CAD build for the part. Positions are in the model's coordinates, mm. A direction names the side the tool comes from. Coordinates: 2 decimals unless noted, no trailing zeros. Order: outer loops, then holes, each group sorted by start corner. A loop starts at its lowest first (then second) coordinate and runs counter-clockwise, first axis right, second up. Notation, with made-up numbers: (-1.5, -28.5) - (16.5, -28.5) arc R26 ccw to (16.5, 6.5) - close; hole circle Ø11 at (-12, 34). An arc over 180 degrees is marked (long way). Use one line per item in the form item = value.
```python
from build123d import *

# Parameters (mm, degrees)
F0_R     = 1
F1_DEPTH = 6.35


with BuildPart() as f1:
    # F0 (on Top) → F1 (new body)
    with BuildSketch(Plane.XY):
        with BuildLine():
            Line((-44.45, 22.732547), (-44.45, -22.6289))
            Line((-44.45, -22.6289), (5.08, -22.6289))
            Line((5.08, -22.6289), (5.08, -17.8029))
            Line((5.08, -17.8029), (9.652, -17.8029))
            Line((9.652, -17.8029), (9.652, -22.248723))
            ThreePointArc((9.652, -22.248723), (32.178133, 0.241912), (9.652, 22.732547))
            Line((9.652, 22.732547), (9.652, 17.906547))
            Line((9.652, 17.906547), (5.08, 17.906547))
            Line((5.08, 17.906547), (5.08, 22.732547))
            Line((5.08, 22.732547), (-44.45, 22.732547))
        make_face()
        with Locations((-24.760989, 0)):
            Circle(F0_R, mode=Mode.SUBTRACT)
        with Locations((5.589839, 0)):
            Circle(F0_R, mode=Mode.SUBTRACT)
        with Locations((20.59151, 0)):
            Circle(F0_R, mode=Mode.SUBTRACT)
    extrude(amount=F1_DEPTH)


solid = f1.part
```
Item 1: Drop flat-ended pins along their axis: pin 1 (1.4 mm diameter, centred on y = -20.5, z = 2, fed in from +X); pin 2 (1.5 mm diameter, centred on x = 14.5, z = 2, fed in from -Y); pin 3 (2.5 mm diameter, centred on x = 7, z = 2, fed in from -Y). Give the stop position or say it passes through.
Derived:
pin_1 = 19.89
pin_2 = -21.88
pin_3 = -17.8
Item 2: Drill centre lines: line 1 (X direction, y = 20, z = 4); line 2 (X direction, y = -10.5, z = 3.5); line 3 (X direction, y = 7, z = 0.5). Where is each one in solid material? Low to high. Write a range as [from, to].
Derived:
line_1 = [-44.45, 5.08], [9.65, 20.43]
line_2 = [-44.45, 29.45]
line_3 = [-44.45, 31.14]
Item 3: Cut at B-B, the plane y = 0. Write the cut outline in (x, z).
Derived:
outline = (-44.45, 0) - (-25.76, 0) - (-25.76, 6.35) - (-44.45, 6.35) - close; (-23.76, 0) - (4.59, 0) - (4.59, 6.35) - (-23.76, 6.35) - close; (6.59, 0) - (19.59, 0) - (19.59, 6.35) - (6.59, 6.35) - close; (21.59, 0) - (32.18, 0) - (32.18, 6.35) - (21.59, 6.35) - close
Item 4: Two-plate mould, pull along Y, no slides. Class faces 1 (the face through (-23.807, 0.3, 3.131)), 2 (the face through (-20, -22.629, 3)), 3 (the face through (9.652, -20, 3)): +Y half, -Y half, draft (parallel to the pull), parting line (faces both ways), or undercut.
Derived:
face_1 = undercut
face_2 = -Y half
face_3 = draft
Item 5: 3-axis set-ups, long thin cutter, end or side, ignore diameter. For faces 4 (the face through (5.08, -20, 3)), 5 (the face through (7, 17.907, 3)), 6 (the face through (-7, 0, 6.35)): which of +Z, -Z, +X, -X, +Y, -Y reach the whole face in a straight line?
Derived:
face_4 = +Z, -Z, -Y
face_5 = +Z, -Z, +Y
face_6 = +Z, +X, -X, +Y, -Y
Item 6: Cut at C-C, the plane y = 15. Write the cut outline in (x, z).
Derived:
outline = (-44.45, 0) - (26.66, 0) - (26.66, 6.35) - (-44.45, 6.35) - close
Item 7: Cut at A-A, the plane z = 2.25. Write the cut outline in (x, y).
Derived:
outline = (-44.45, -22.63) - (5.08, -22.63) - (5.08, -17.8) - (9.65, -17.8) - (9.65, -22.25) arc R22.49 ccw to (9.65, 22.73) - (9.65, 17.91) - (5.08, 17.91) - (5.08, 22.73) - (-44.45, 22.73) - close; hole circle Ø2 at (-24.76, 0); hole circle Ø2 at (5.59, 0); hole circle Ø2 at (20.59, 0)
Item 8: Cut at D-D, the plane y = -9. Write the cut outline in (x, z), plus the area to 3 significant figures.
Derived:
outline = (-44.45, 0) - (30.19, 0) - (30.19, 6.35) - (-44.45, 6.35) - close
area = 474 mm²
